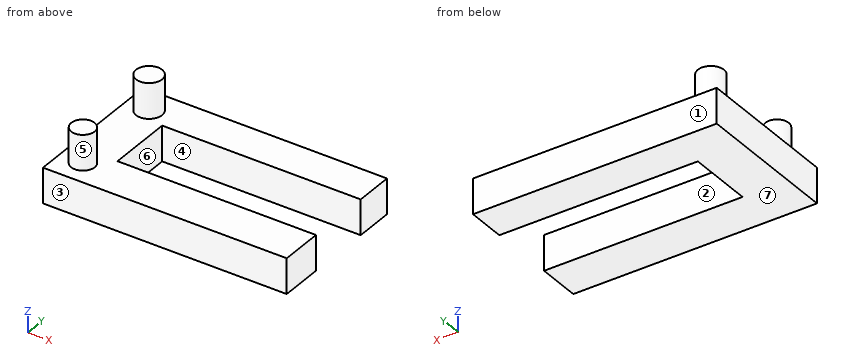
from build123d import *

# Parameters (mm, degrees)
F1_DEPTH = 25.4
F2_R     = 9.414196
F2_R_2   = 8.478638
F3_DEPTH = 25.4


with BuildPart() as f1:
    # F0 (on Top) → F1 (new body)
    with BuildSketch(Plane.XY):
        Polygon((0, 105.842702), (0, 0), (175.859332, 0), (175.859332, 30.87078), (32.630205, 30.87078), (32.630205, 78.058995), (175.859332, 78.058995), (175.859332, 105.842702), align=None)
    extrude(amount=F1_DEPTH)

    # F2 (on face) → F3 (join)
    with BuildSketch(Plane.XY.offset(25.4)):
        with Locations((16.756006, 87.473191)):
            Circle(F2_R)
        with Locations((16.756006, 17.66476)):
            Circle(F2_R_2)
    extrude(amount=F3_DEPTH)


solid = f1.part
Work out the finished part from the listing and answer in its coordinate system (mm). Face numbers are marked on the shaded views. A direction names the side the tool comes from. Give positions to 0.01 mm unless a question says otherwise; leave off trailing zeros. Loops run counter-clockwise (first coordinate to the right, second up) from the corner with the lowest first, then second, coordinate; pieces in that order, holes last. Notation, with made-up numbers: (-30, 10) - (-16, 10) arc R27 cw to (-16, 48) - close; hole circle Ø2 at (78, -12). An arc over 180 degrees is marked (long way). Answer in a Markdown table with one row per item.
(1) Section C-C (y = 83) is taken. Give the vertices of the cut face in (x, z), and give its area (3 significant figures).
Results list:
| item | result |
|---|---|
| outline | (0, 0) - (175.86, 0) - (175.86, 25.4) - (25.04, 25.4) - (25.04, 50.8) - (8.47, 50.8) - (8.47, 25.4) - (0, 25.4) - close |
| area | 4,890 mm² |
(2) Section B-B (z = 12) is taken. Give the vertices of the cut face in (x, y).
Results list:
| item | result |
|---|---|
| outline | (0, 0) - (175.86, 0) - (175.86, 30.87) - (32.63, 30.87) - (32.63, 78.06) - (175.86, 78.06) - (175.86, 105.84) - (0, 105.84) - close |
(3) Section D-D (z = 33) is taken. Give the vertices of the cut face in (x, y).
Results list:
| item | result |
|---|---|
| outline | circle Ø18.83 at (16.76, 87.47); circle Ø16.96 at (16.76, 17.66) |
(4) Flat-ended cylindrical pins translate along their axes: pin 1 Ø7.5 at (y, z) = (65.5, 15) entering from +X; pin 2 Ø20.5 at (x, z) = (85, 18.5) entering from -Y; pin 3 Ø8 at (x, y) = (75, 30) entering from +Z. Find the tip coordinate at first contact, or state that the pin passes through.
Results list:
| item | result |
|---|---|
| pin 1 | stops at x = 32.63 |
| pin 2 | stops at y = 0 |
| pin 3 | stops at z = 25.4 |
(5) Section A-A (x = 76) is taken. Give the vertices of the cut face in (y, z), and give its area (3 significant figures).
Results list:
| item | result |
|---|---|
| outline | (0, 0) - (30.87, 0) - (30.87, 25.4) - (0, 25.4) - close; (78.06, 0) - (105.84, 0) - (105.84, 25.4) - (78.06, 25.4) - close |
| area | 1,490 mm² |
(6) Consider L1, parallel to Y at x = 108.5, z = 21; L2, parallel to Z at x = 164, y = 93; L3, parallel to X at y = 58, z = 17. Determine where each line is inside the solid, lowest interval first. Write a range as [from, to].
Results list:
| item | result |
|---|---|
| L1 | y = [0, 30.87], [78.06, 105.84] |
| L2 | z = [0, 25.4] |
| L3 | x = [0, 32.63] |
(7) For a pull along Y with two mould halves and no side action, classify the marked faces 1, 2, 3 and 4 as pulls with the +Y half, pulls with the -Y half, needs draft (parallel to the pull), parting line crosses it, or undercut.
Results list:
| item | result |
|---|---|
| face 1 | pulls with the +Y half |
| face 2 | undercut |
| face 3 | pulls with the -Y half |
| face 4 | undercut |
(8) A tool of negligible diameter and unlimited length cuts with its end or side. For the marked faces 5, 6 and 7, from which of +Z, -Z, +X, -X, +Y, -Y can it reach the whole face along a straight path? Write none if from no direction.
Results list:
| item | result |
|---|---|
| face 5 | +Z |
| face 6 | +Z, -Z, +X |
| face 7 | -Z, +X, -X, +Y, -Y |
